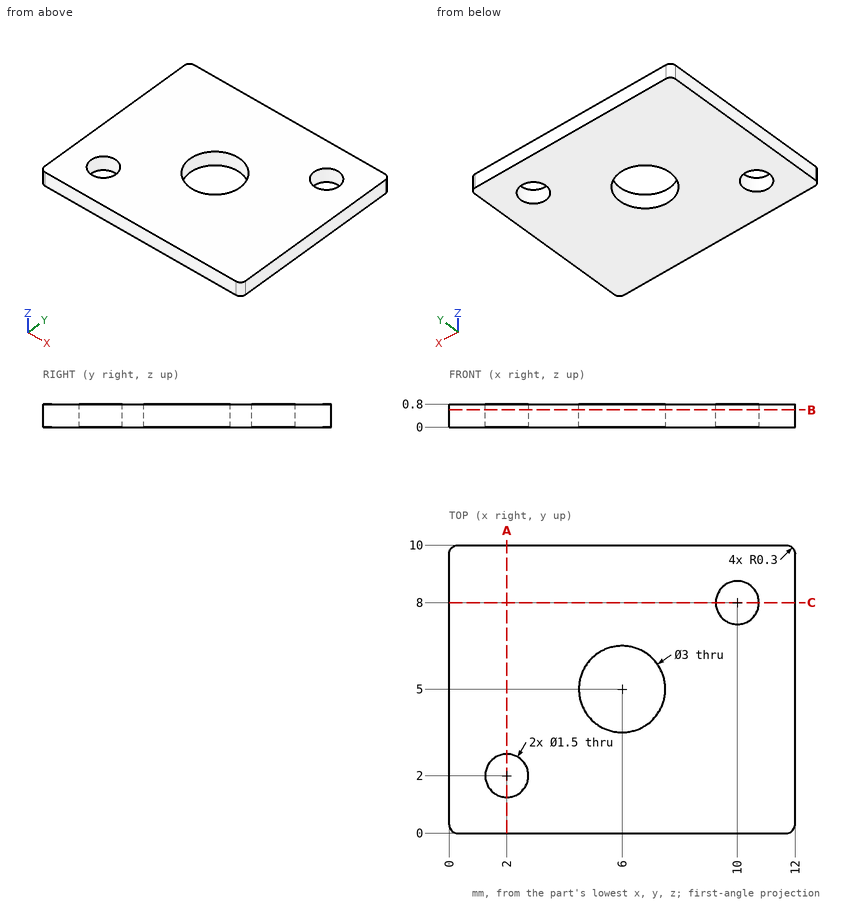
The figure shows three views and two pictorial views of one solid part (mm, origin at its lowest corner). Answer the questions. Give positions to 0.01 mm unless a question says otherwise; leave off trailing zeros. Loops run counter-clockwise (first coordinate to the right, second up) from the corner with the lowest first, then second, coordinate; pieces in that order, holes last. Notation, with made-up numbers: (82, 81) -> (86, 81) arc R31 cw to (86, 114) -> close; hole circle Ø4 at (56, -24.75). An arc over 180 degrees is marked (long way). Use a Markdown table: item, result. Add a question column.
1. Find the intervals of material crossed by probe 1 along Y at (x, z) = (10, 0.1); probe 2 along Y at (x, z) = (6, 0.45); probe 3 along X at (y, z) = (4.5, 0.5), in increasing order.
2. Section C-C on y = 8 is taken. Determine the outline of the cut face in (x, z).
3. Section A-A on x = 2 is taken. Determine the outline of the cut face in (y, z), and give its area (3 significant figures).
4. Section B-B on z = 0.6 is taken. Determine the outline of the cut face in (x, y), and give its area (3 significant figures).
Results below:
| question | item | result |
|---|---|---|
| 1 | probe 1 | y = 0 to 7.25, 8.75 to 10 |
| 1 | probe 2 | y = 0 to 3.5, 6.5 to 10 |
| 1 | probe 3 | x = 0 to 4.59, 7.41 to 12 |
| 2 | outline | (0, 0) -> (9.25, 0) -> (9.25, 0.8) -> (0, 0.8) -> close; (10.75, 0) -> (12, 0) -> (12, 0.8) -> (10.75, 0.8) -> close |
| 3 | outline | (0, 0) -> (1.25, 0) -> (1.25, 0.8) -> (0, 0.8) -> close; (2.75, 0) -> (10, 0) -> (10, 0.8) -> (2.75, 0.8) -> close |
| 3 | area | 6.80 mm^2 |
| 4 | outline | (0, 0.3) arc R0.3 ccw to (0.3, 0) -> (11.7, 0) arc R0.3 ccw to (12, 0.3) -> (12, 9.7) arc R0.3 ccw to (11.7, 10) -> (0.3, 10) arc R0.3 ccw to (0, 9.7) -> close; hole circle Ø1.5 at (2, 2); hole circle Ø3 at (6, 5); hole circle Ø1.5 at (10, 8) |
| 4 | area | 109 mm^2 |
